Autodesk Inventor part; units mm, degrees
ref_plane "bolt_XY" through (0, 0, 0) normal (1, 0, 0) x (0, 0, -1)
ref_plane "bolt_YZ" through (0, 0, 0) normal (0, 0, -1) x (0, 1, 0)
ref_plane "bolt_ZX" through (0, 0, 0) normal (0, 1, 0) x (1, 0, 0)
sketch "Sketch_1" plane through (0, 0, 0) normal (0, 0, 1) x (1, 0, 0)
  line L0 (23.25, 0) -> (-5.5, 0)
  line L1 (-5.5, 0) -> (-5.5, 5.95)
  line L2 (-5.5, 5.95) -> (-4.85, 6.6)
  line L3 (-4.85, 6.6) -> (0, 6.6)
  line L4 (0, 6.6) -> (0, 3.71)
  line L5 (0, 3.71) -> (2.246, 3.71)
  arc A0 (2.246, 3.71) -> (2.4983, 3.9935) centre (2.246, 3.964) ccw
  line L6 (2.4983, 3.9935) -> (12, 3.9935)
  line L7 (12, 3.9935) -> (12, 2.708)
  arc A1 (12, 2.708) -> (12.508, 2.2) centre (12.508, 2.708) ccw
  line L8 (12.508, 2.2) -> (14.346, 2.2)
  arc A2 (14.346, 2.2) -> (14.6, 2.454) centre (14.346, 2.454) ccw
  line L9 (14.6, 2.454) -> (14.6, 3)
  line L10 (14.6, 3) -> (22.6365, 3)
  line L11 (22.6365, 3) -> (23.25, 2.3865)
  line L12 (23.25, 2.3865) -> (23.25, 0)
  line L13 (23.25, 0) -> (-5.5, 0)
revolve "Revolution1" add sketch "Sketch_1" angle 360 about axis through (23.25, 0, 0) along (1, 0, 0)
thread "Thread1"
sketch "Sketch_5" plane through (-5.5, 0, 0) normal (1, 0, 0) x (0, 0, -1)
  line L0 (-2.042, -1.1789) -> (0, -2.3579)
  line L1 (0, -2.3579) -> (2.042, -1.1789)
  line L2 (2.042, -1.1789) -> (2.042, 1.1789)
  line L3 (2.042, 1.1789) -> (0, 2.3579)
  line L4 (0, 2.3579) -> (-2.042, 1.1789)
  line L5 (-2.042, 1.1789) -> (-2.042, -1.1789)
extrude "Extrusion1" cut sketch "Sketch_5" along normal blind 3.3
ref_plane "bolt_XY" through (0, 0, 0) normal (1, 0, 0) x (0, 0, -1)
ref_plane "bolt_YZ" through (0, 0, 0) normal (0, 0, -1) x (0, 1, 0)
ref_plane "bolt_ZX" through (0, 0, 0) normal (0, 1, 0) x (1, 0, 0)
ref_plane "bolt1_XY" through (15.2, 0, 0) normal (1, 0, 0) x (0, 0, -1)
ref_plane "bolt1_YZ" through (15.2, 0, 0) normal (0, 0, -1) x (0, 1, 0)
ref_plane "bolt1_ZX" through (15.2, 0, 0) normal (0, 1, 0) x (1, 0, 0)
properties part number "25-2281_b"
Input: part model. Units: mm. Frame: model coordinates. A direction names the side the tool comes from. Give positions to 0.01 mm unless a question says otherwise; leave off trailing zeros. Write each loop counter-clockwise with the first axis right and the second up, starting at its lowest first coordinate (ties: lowest second). Pieces come first, ordered by that corner, then holes. Notation, with made-up numbers: M 6.25,-34.75 L 39.25,-34.75 A21 ccw 39.25,-7.75 Z; hole C 58.5,78 d2. An arc over 180 degrees is marked long. Use one line per item in the form item = value.
1. Cut plane B-B on x = 4.25. Return loops of the section in (y, z).
Outcome:
outline = C 0,0 d7.99
2. Mould query, pull axis Y, two halves, no side actions, for faces 1 (the face through (-3.873, 1.76, -1.035)), 2 (the face through (0, 3, -3)), 3 (the face through (-2.391, -4.864, 4.461)), 4 (the face through (-3.873, -1.777, -1.007)). Classes: released by +Y, released by -Y, zero draft, split by the parting line, or undercut.
Outcome:
face_1 = undercut
face_2 = zero draft
face_3 = split by the parting line
face_4 = undercut
3. Cut plane C-C on x = 20. Return loops of the section in (y, z), and give its area (3 significant figures).
Outcome:
outline = C 0,0 d6
area = 28.3 mm²
4. Ray query, L1, parallel to X at y = -0.25, z = 1.25; L2, parallel to X at y = -1.5, z = -4.75; L3, parallel to X at y = -2, z = -1.5. Return the intervals inside material, ascending.
Outcome:
L1 = -2.2 to 23.25
L2 = -5.5 to 0
L3 = -5.5 to 12.04, 14.6 to 23.14
5. First-contact query: P1, Ø1, axis at x = 11.5, z = 3.5, coming from the +Y side; P2, Ø4, axis at x = 5, y = 3, coming from the +Z side; P3, Ø1.5, axis at x = 12, z = -3.5, coming from the -Y side. Flat tips, straight axial feed; report the tip coordinate or a pass-through.
Outcome:
P1 = 2.64
P2 = 3.87
P3 = -2.9
6. Reachability of faces 5 (the face through (7.32, -2.94, 2.7)), 6 (the face through (-4, 0, 2.042)), 7 (the face through (-5.5, 3, 0)), 8 (the face through (13.44, 2.1, 0.66)) from +Z, -Z, +X, -X, +Y, -Y: full face, straight path, thin tool, end or side. Return the list, or none.
Outcome:
face_5 = +X
face_6 = -X
face_7 = +Z, -Z, -X, +Y, -Y
face_8 = none
